```python
from build123d import *

# Parameters (mm, degrees)
F0_R     = 6.35
F1_DEPTH = 12.7
F2_DEPTH = 5.08
F3_DEPTH = 101.6


with BuildPart() as f1:
    # F0 (on Front) → F1 (new body)
    with BuildSketch(Plane.XZ):
        with BuildLine():
            ThreePointArc((152.4, 0), (146.674755, 16.064371), (132.08, 24.886816))
            ThreePointArc((132.08, 24.886816), (101.6, 0), (132.08, -24.886816))
            ThreePointArc((132.08, -24.886816), (146.674755, -16.064371), (152.4, 0))
        make_face()
        with Locations((127, 0)):
            Circle(F0_R, mode=Mode.SUBTRACT)
        with BuildLine():
            ThreePointArc((10.16, -49.773632), (39.349511, -32.128741), (50.8, 0))
            ThreePointArc((50.8, 0), (39.349511, 32.128741), (10.16, 49.773632))
            ThreePointArc((10.16, 49.773632), (-50.8, 0), (10.16, -49.773632))
        make_face()
        Circle(F0_R, mode=Mode.SUBTRACT)
    extrude(amount=F1_DEPTH)

    # F0 (on Front) → F2 (join)
    with BuildSketch(Plane.XZ):
        with BuildLine():
            ThreePointArc((10.16, 49.773632), (39.349511, 32.128741), (50.8, 0))
            ThreePointArc((50.8, 0), (39.349511, -32.128741), (10.16, -49.773632))
            Line((10.16, -49.773632), (132.08, -24.886816))
            ThreePointArc((132.08, -24.886816), (101.6, 0), (132.08, 24.886816))
            Line((132.08, 24.886816), (10.16, 49.773632))
        make_face()
    extrude(amount=F2_DEPTH)

    # F0 (on Front) → F3 (cut)
    with BuildSketch(Plane.XZ):
        Circle(F0_R)
    extrude(amount=F3_DEPTH, mode=Mode.SUBTRACT)


solid = f1.part
```
Geometry check sheet. Reference: the model listing, model coordinates, mm. Give positions to 0.01 mm unless a question says otherwise; leave off trailing zeros. Loops run counter-clockwise (first coordinate to the right, second up) from the corner with the lowest first, then second, coordinate; pieces in that order, holes last. Notation, with made-up numbers: (9.5, 64.5) - (18.5, 64.5) arc R11 cw to (18.5, 69.5) - close; hole circle Ø4 at (45.5, 28). An arc over 180 degrees is marked (long way). Use CSV: the item, a comma, the result in double quotes. Start each with the question number.
Q1. Go/stop test with flat-tipped pins: pin 1 Ø4 at (y, z) = (-1.5, -9) entering from +X; pin 2 Ø5 at (x, y) = (-7.5, -1.5) entering from +Z; pin 3 Ø1.5 at (y, z) = (-6, -39) entering from -X. Record where each tip stops, or that it passes through.
Q2. Scan lines: probe 1 along Z at (x, y) = (127, -7); probe 2 along Z at (x, y) = (0, -8); probe 3 along Y at (x, z) = (40.5, -40). Record each from-to range of solid material in increasing order. Write a range as from..to.
Q3. Section check D-D, the plane x = 127. Record the cut outline in (y, z), and give its area (3 significant figures).
Q4. Section check B-B, the plane x = 0. Record the cut outline in (y, z), and give its area (3 significant figures).
Q5. Section check A-A, the plane y = -9. Record the cut outline in (x, z), and give its area (3 significant figures).
Q6. Release check for a two-part mould opening along X. For faces 1 (the face through (11, -12.7, 1)), 2 (the face through (-1.38, -6.26, -6.2)), 3 (the face through (70.267, -2.504, -37.504)) record: +X half, -X half, draft (parallel to the pull), parting line (faces both ways), or undercut.
Q7. Section check C-C, the plane z = -44. Record the cut outline in (x, y), and give its area (3 significant figures).
Findings below:
1,pin 1,"stops at x = 151.42"
1,pin 2,"stops at z = 50.55"
1,pin 3,"stops at x = -33.43"
2,probe 1,"z = -25.4..-6.35, 6.35..25.4"
2,probe 2,"z = -50.8..-6.35, 6.35..50.8"
2,probe 3,"y = -5.08..0"
3,outline,"(-12.7, -25.4) - (-5.08, -25.4) - (-5.08, -25.92) - (0, -25.92) - (0, -6.35) - (-12.7, -6.35) - close; (-12.7, 6.35) - (0, 6.35) - (0, 25.92) - (-5.08, 25.92) - (-5.08, 25.4) - (-12.7, 25.4) - close"
3,area,"489 mm^2"
4,outline,"(-12.7, -50.8) - (0, -50.8) - (0, -6.35) - (-12.7, -6.35) - close; (-12.7, 6.35) - (0, 6.35) - (0, 50.8) - (-12.7, 50.8) - close"
4,area,"1,130 mm^2"
5,outline,"circle Ø101.6 at (0, 0); circle Ø50.8 at (127, 0); hole circle Ø12.7 at (0, 0); hole circle Ø12.7 at (127, 0)"
5,area,"9,880 mm^2"
6,face 1,"draft"
6,face 2,"undercut"
6,face 3,"+X half"
7,outline,"(-25.39, -12.7) - (25.39, -12.7) - (25.39, -5.08) - (38.44, -5.08) - (38.44, 0) - (-25.39, 0) - close"
7,area,"711 mm^2"
